Input: part model. Units: mm. Frame: model coordinates. A direction names the side the tool comes from. Round coordinates to 2 decimals unless told otherwise and drop trailing zeros. Loops run counter-clockwise (first coordinate to the right, second up) from the corner with the lowest first, then second, coordinate; pieces in that order, holes last.
(1) Line query: line 1 (Z direction, x = -90.8, y = 3.85); line 2 (Y direction, x = -25, z = -73.5); line 3 (X direction, y = 1.45, z = -70.8) (3 decimals). Output: solid intervals per line, ascending.
(2) Cut plane C-C, the plane y = 3.65. Output: boundary loops of the cut face in (x, z).
(3) Cut plane B-B, the plane z = -70.8. Output: boundary loops of the cut face in (x, y) (3 decimals).
(4) Draft query along X for faces 1 (the face through (-4, 5, -71)), 2 (the face through (-89, 2, -4)), 3 (the face through (-93, 1, -44)). Return one class per face: released by +X, released by -X, zero draft, split by the parting line, or undercut.
(5) Access query for faces 4 (the face through (-86.8, 3.5, -4.6)), 5 (the face through (-4, 2, -4)), 6 (the face through (-91.606, 3.479, -5.765)). Directions: +Z, -Z, +X, -X, +Y, -Y. A direction counts if a zero-diameter tool reaches every point of the face in a straight line with its end or side. Return the directions, or none.
(6) Cut plane D-D, the plane x = -51. Output: boundary loops of the cut face in (y, z).
(7) First-contact query: pin 1 Ø1.6 at (x, z) = (-90, -71.5) entering from -Y; pin 2 Ø1 at (x, z) = (-31.5, -38.5) entering from +Y. Flat tips, straight axial feed; report the tip coordinate or a pass-through.
(8) Cut plane A-A, the plane x = -2.2. Output: boundary loops of the cut face in (y, z) (3 decimals).
Autodesk Inventor part; units mm, degrees
ref_plane "YZ Plane" through (0, 0, 0) normal (1, 0, 0) x (0, 1, 0)
ref_plane "XZ Plane" through (0, 0, 0) normal (0, 1, 0) x (-1, 0, 0)
ref_plane "XY Plane" through (0, 0, 0) normal (0, 0, 1) x (1, 0, 0)
sketch "Sketch1" plane through (0, 0, 0) normal (0, 1, 0) x (-1, 0, 0)
  line L0 (0, 0) -> (93, 0)
  line L1 (93, 0) -> (93, -90)
  line L2 (93, -90) -> (0, -90)
  line L3 (0, -90) -> (0, 0)
  circle A0 centre (90.8, -4.5) radius 1.5
  circle A1 centre (90.8, -70.8) radius 1.5
  circle A2 centre (2.2, -4.5) radius 1.5
  circle A3 centre (2.2, -70.8) radius 1.5
  arc A4 (0, -74.1407) -> (0, -67.4593) centre (2.2, -70.8) ccw
  arc A5 (0, -7.8407) -> (0, -1.1593) centre (2.2, -4.5) ccw
  arc A6 (93, -67.4593) -> (93, -74.1407) centre (90.8, -70.8) ccw
  arc A7 (93, -1.1593) -> (93, -7.8407) centre (90.8, -4.5) ccw
  dimension "d0" = 93
  dimension "d1" = 90
  dimension "d13" = 3
  dimension "d14" = 3
  dimension "d15" = 3
  dimension "d39" = 8
  dimension "d40" = 8
  dimension "d41" = 8
  dimension "d42" = 8
extrude "Extrusion6" add sketch "Sketch1" along normal blind 2 contours L0 L1 A7 A6 L2 L3 A4 A5
extrude "Extrusion7" add sketch "Sketch1" along normal blind 5 contours A5 L3 | L1 A7 | A4 L3 | L1 A6
sketch "Sketch4" plane through (0, 0, 0) normal (0, -1, 0) x (1, 0, 0)
  circle A0 centre (-2.2, -4.5) radius 1.5
  circle A1 centre (-2.2, -4.5) radius 3.125
  circle A2 centre (-2.2, -70.8046) radius 3.125
  circle A3 centre (-90.8, -4.5) radius 1.5
  circle A4 centre (-90.8, -4.5) radius 3.125
  circle A5 centre (-90.8, -70.8) radius 1.5
  circle A6 centre (-90.8, -70.8) radius 3.125
  point P0 (0, 0)
  dimension "d47" = 6.25
  dimension "d48" = 6.25
  dimension "d49" = 6.25
  dimension "d50" = 6.25
extrude "Extrusion8" cut sketch "Sketch4" against normal blind 2 contours A0 | A1 | A2 | A4 | A5 | A6
properties part number "caseBack"
Reported:
1. line 1: z = -74.8 to -72.3, -69.3 to -66.8, -8.5 to -6, -3 to -0.5
1. line 2: y = 0 to 2
1. line 3: x = -87.675 to -5.325
2. outline: (-93, -74.14) arc R4 ccw (long way) to (-93, -67.46) - close; (-93, -7.84) arc R4 ccw (long way) to (-93, -1.16) - close; (0, -74.14) - (0, -67.46) arc R4 ccw (long way) to start; (0, -7.84) - (0, -1.16) arc R4 ccw (long way) to start; hole circle Ø3 at (-90.8, -70.8); hole circle Ø3 at (-90.8, -4.5); hole circle Ø3 at (-2.2, -70.8); hole circle Ø3 at (-2.2, -4.5)
3. outline: (-93, 2) - (-92.3, 2) - (-92.3, 5) - (-93, 5) - close; (-89.3, 2) - (-87.675, 2) - (-87.675, 0) - (-5.325, 0) - (-5.325, 2) - (-3.7, 2) - (-3.7, 5) - (-6.2, 5) - (-6.2, 2) - (-86.8, 2) - (-86.8, 5) - (-89.3, 5) - close; (-0.7, 2) - (0, 2) - (0, 5) - (-0.7, 5) - close
4. face 1: zero draft
4. face 2: undercut
4. face 3: released by -X
5. face 4: +Y
5. face 5: -Y
5. face 6: +Y, -Y
6. outline: (0, -90) - (2, -90) - (2, 0) - (0, 0) - close
7. pin 1: stops at y = 2
7. pin 2: stops at y = 2
8. outline: (0, -90) - (2, -90) - (2, -74.8) - (5, -74.8) - (5, -72.3) - (2, -72.3) - (2, -73.93) - (0, -73.93) - close; (0, -67.68) - (2, -67.68) - (2, -69.3) - (5, -69.3) - (5, -66.8) - (2, -66.8) - (2, -8.5) - (5, -8.5) - (5, -6) - (2, -6) - (2, -7.625) - (0, -7.625) - close; (0, -1.375) - (2, -1.375) - (2, -3) - (5, -3) - (5, -0.5) - (2, -0.5) - (2, 0) - (0, 0) - close
